Design review of the part built by this model. Coordinates are the model's own, in mm. A direction names the side the tool comes from. Coordinates: 2 decimals unless noted, no trailing zeros. Write each loop counter-clockwise with the first axis right and the second up, starting at its lowest first coordinate (ties: lowest second). Pieces come first, ordered by that corner, then holes. Notation, with made-up numbers: (-3, -11) -> (11, -11) arc R19 ccw to (11, 1) -> close; hole circle Ø4 at (1.5, -23). An arc over 180 degrees is marked (long way). Answer in a Markdown table with one row per item. Add a question column.
Item 1: Take a section at A-A, the plane z = 19. Write out the cut boundary in (x, y), and give its area (3 significant figures).
Item 2: For faces 1 (the face through (0, 7, 49)), 2 (the face through (-23, -32, 49)), 3 (the face through (-27, -27, 49)), list the 3-axis set-ups (+Z, -Z, +X, -X, +Y, -Y) from which the entire face can be reached by the end or side of a thin tool; tool diameter is ignored.
Item 3: Take a section at B-B, the plane y = -4. Write out the cut boundary in (x, z).
Item 4: Clearance check with flat-ended pins moving along their axes: P1, Ø1.5, axis at x = -21.5, z = 43, coming from the +Y side; P2, Ø12.5, axis at y = -1.5, z = 44, coming from the -X side. State where each tip first meets the part, or that it passes through.
Item 5: Take a section at C-C, the plane x = -32. Write out the cut boundary in (y, z).
Item 6: To check wall thickness, follow line 1 (Y direction, x = -41, z = 48); line 2 (X direction, y = -26, z = 47); line 3 (X direction, y = 8, z = 34). State the ranges of each line that lie inside material, in increasing order.
from build123d import *

# Parameters (mm, degrees)
F0_W     = 5
F0_H     = 15
F0_H_2   = 5
F1_DEPTH = 100
F2_DEPTH = 27
F3_DEPTH = 27


with BuildPart() as f1:
    # F0 (on Top) → F1 (new body)
    with BuildSketch(Plane.XY):
        Polygon((0, -5), (0, 0), (-5, 0), (-50, 0), (-50, -5), align=None)
        with Locations((-2.5, 7.5)):
            Rectangle(F0_W, F0_H)
        with Locations((2.5, -2.5)):
            Rectangle(F0_W, F0_H_2)
    extrude(amount=F1_DEPTH)

    # F2 (add): a face of the model
    f2_faces = [f1.faces().sort_by_distance(p)[0] for p in [
        (-22.5, -5, 50),
    ]]
    extrude(f2_faces, amount=F2_DEPTH)

    # F3 (cut): a face of the model
    f3_faces = [f1.faces().sort_by_distance(p)[0] for p in [
        (-27.5, 0, 50),
    ]]
    extrude(f3_faces, amount=-F3_DEPTH, mode=Mode.SUBTRACT)


solid = f1.part
Answers:
| question | item | result |
|---|---|---|
| 1 | outline | (-50, -32) -> (5, -32) -> (5, 0) -> (0, 0) -> (0, 15) -> (-5, 15) -> (-5, -27) -> (-50, -27) -> close |
| 1 | area | 620 mm^2 |
| 2 | face 1 | +Z, -Z, +X, +Y |
| 2 | face 2 | +Z, -Z, +X, -X, -Y |
| 2 | face 3 | +Z, -Z, -X, +Y |
| 3 | outline | (-5, 0) -> (5, 0) -> (5, 100) -> (-5, 100) -> close |
| 4 | P1 | stops at y = -27 |
| 4 | P2 | stops at x = -5 |
| 5 | outline | (-32, 0) -> (-27, 0) -> (-27, 100) -> (-32, 100) -> close |
| 6 | line 1 | y = -32 to -27 |
| 6 | line 2 | x = -5 to 5 |
| 6 | line 3 | x = -5 to 0 |
